Read the model definition and answer for the solid it produces. Units are mm, in the model's axes. A direction names the side the tool comes from. Coordinates: 2 decimals unless noted, no trailing zeros. Loops run counter-clockwise (first coordinate to the right, second up) from the corner with the lowest first, then second, coordinate; pieces in that order, holes last. Notation, with made-up numbers: (-26, 73) - (-19, 73) arc R30 ccw to (-19, 99) - close; hole circle Ø6 at (15.5, 73.5). An arc over 180 degrees is marked (long way). Use one line per item in the form item = value.
from build123d import *

# Parameters (mm, degrees)
CROQUIS1_W               = 118
CROQUIS1_H               = 74
SALIENTE_EXTRUIR1_DEPTH  = 5
CROQUIS2_W               = 50
CROQUIS2_H               = 40
CORTAR_EXTRUIR1_DEPTH    = 5
CROQUIS3_W               = 50
CROQUIS3_H               = 5
SALIENTE_EXTRUIR2_DEPTH  = 3
CROQUIS4_W               = 4.8
CROQUIS4_H               = 2.8
CROQUIS4_W_2             = 2.8
CROQUIS4_H_2             = 4.8
CORTAR_EXTRUIR2_DEPTH    = 6
CROQUIS5_W               = 3
CROQUIS5_H               = 40
CORTAR_EXTRUIR3_DEPTH    = 3
CROQUIS6_W               = 12
CROQUIS6_H               = 40
SALIENTE_EXTRUIR3_DEPTH  = 40
CROQUIS8_W               = 4
CROQUIS8_H               = 35
SALIENTE_EXTRUIR5_DEPTH  = 5
SALIENTE_EXTRUIR7_DEPTH  = 33
CORTAR_EXTRUIR6_DEPTH    = 11
CORTAR_EXTRUIR7_DEPTH    = 13
CORTAR_EXTRUIR8_DEPTH    = 13
CORTAR_EXTRUIR9_DEPTH    = 11
CROQUIS10_W              = 1.9
CROQUIS10_H              = 35
SALIENTE_EXTRUIR9_DEPTH  = 8
CROQUIS22_W              = 3.1
CROQUIS22_H              = 35
SALIENTE_EXTRUIR10_DEPTH = 2
CORTAR_EXTRUIR11_DEPTH   = 40
CROQUIS23_W              = 3
CROQUIS23_H              = 40
SALIENTE_EXTRUIR11_DEPTH = 10
CORTAR_EXTRUIR12_DEPTH   = 10
CORTAR_EXTRUIR13_DEPTH   = 10
CORTAR_EXTRUIR14_DEPTH   = 40
CROQUIS28_R              = 1.25
CORTAR_EXTRUIR15_DEPTH   = 5
SALIENTE_EXTRUIR12_DEPTH = 37
CROQUIS30_W              = 29.42787794
CROQUIS30_H              = 11
SALIENTE_EXTRUIR13_DEPTH = 1.970920231
CHAFL_N1_SIZE            = 5
CHAFL_N1_SIZE2           = 18
CHAFL_N2_SIZE            = 5
CHAFL_N2_SIZE_2          = 13
CHAFL_N3_SIZE            = 5
CHAFL_N3_SIZE_2          = 13
CROQUIS51_W              = 8
CROQUIS51_H              = 14
CORTAR_EXTRUIR23_DEPTH   = 10
CROQUIS52_W              = 9
CROQUIS52_H              = 11
CROQUIS52_W_2            = 8
CROQUIS52_W_3            = 4.539822883
CORTAR_EXTRUIR25_DEPTH   = 10
SALIENTE_EXTRUIR20_DEPTH = 12
CROQUIS54_W              = 5
CROQUIS54_H              = 11
CORTAR_EXTRUIR26_DEPTH   = 10
CROQUIS55_W              = 5
CROQUIS55_H              = 11
CORTAR_EXTRUIR30_DEPTH   = 10


with BuildPart() as part:
    # Croquis1 → Saliente-Extruir1 (new body)
    with BuildSketch(Plane.XY):
        Rectangle(CROQUIS1_W, CROQUIS1_H)
    extrude(amount=SALIENTE_EXTRUIR1_DEPTH)

    # Croquis2 → Cortar-Extruir1 (cut)
    with BuildSketch(Plane.XY.offset(5)):
        with Locations((-21, 0)):
            Rectangle(CROQUIS2_W, CROQUIS2_H)
    extrude(amount=-CORTAR_EXTRUIR1_DEPTH, mode=Mode.SUBTRACT)

    # Croquis3 → Saliente-Extruir2 (add)
    with BuildSketch(Plane.XY.offset(5)):
        with Locations((34, 34.5)):
            Rectangle(CROQUIS3_W, CROQUIS3_H)
        with Locations((34, -34.5)):
            Rectangle(CROQUIS3_W, CROQUIS3_H)
    extrude(amount=SALIENTE_EXTRUIR2_DEPTH)

    # Croquis4 → Cortar-Extruir2 (cut)
    with BuildSketch(Plane.XY.offset(8)):
        with Locations((54.5, 34.5)):
            Rectangle(CROQUIS4_W, CROQUIS4_H)
        with Locations((12.5, 34.5)):
            Rectangle(CROQUIS4_W, CROQUIS4_H)
        with Locations((12.5, -34.5)):
            Rectangle(CROQUIS4_W, CROQUIS4_H)
        with Locations((54.5, -34.5)):
            Rectangle(CROQUIS4_W, CROQUIS4_H)
        with Locations((-56.5, -32.5)):
            Rectangle(CROQUIS4_W_2, CROQUIS4_H_2)
        with Locations((-56.5, 32.5)):
            Rectangle(CROQUIS4_W_2, CROQUIS4_H_2)
    extrude(amount=-CORTAR_EXTRUIR2_DEPTH, mode=Mode.SUBTRACT)

    # Croquis5 → Cortar-Extruir3 (cut)
    with BuildSketch(Plane.XY.offset(5)):
        with Locations((39.5, 0)):
            Rectangle(CROQUIS5_W, CROQUIS5_H)
    extrude(amount=-CORTAR_EXTRUIR3_DEPTH, mode=Mode.SUBTRACT)

    # Croquis6 → Saliente-Extruir3 (add)
    with BuildSketch(Plane.XY.offset(2)):
        with Locations((47, 0)):
            Rectangle(CROQUIS6_W, CROQUIS6_H)
    extrude(amount=SALIENTE_EXTRUIR3_DEPTH)

    # Croquis8 → Saliente-Extruir5 (add)
    with BuildSketch(Plane.XY.offset(5)):
        with Locations((15, 0)):
            Rectangle(CROQUIS8_W, CROQUIS8_H)
    extrude(amount=SALIENTE_EXTRUIR5_DEPTH)

    # Croquis12 → Saliente-Extruir7 (add)
    with BuildSketch(Plane.XY.offset(5)):
        Polygon((26, -19), (38, -19), (38, -32), (31, -32), (31, -21), (26, -21), align=None)
        Polygon((31, 32), (38, 32), (38, 19), (26, 19), (26, 21), (31, 21), align=None)
    extrude(amount=SALIENTE_EXTRUIR7_DEPTH)

    # Croquis14 → Cortar-Extruir6 (cut)
    with BuildSketch(Plane(origin=(0, 32, 0), x_dir=(1, 0, 0), z_dir=(0, 1, 0))):
        Polygon((31, -38), (36, -38), (31, -9), align=None)
    extrude(amount=-CORTAR_EXTRUIR6_DEPTH, mode=Mode.SUBTRACT)

    # Croquis16 → Cortar-Extruir7 (cut)
    with BuildSketch(Plane.XZ.offset(-19)):
        Polygon((38, 38), (38, 5), (33, 5), (33, 9), align=None)
    extrude(amount=-CORTAR_EXTRUIR7_DEPTH, mode=Mode.SUBTRACT)

    # Croquis17 → Cortar-Extruir8 (cut)
    with BuildSketch(Plane.XZ.offset(32)):
        Polygon((38, 38), (38, 5), (33, 5), (33, 9), align=None)
    extrude(amount=-CORTAR_EXTRUIR8_DEPTH, mode=Mode.SUBTRACT)

    # Croquis18 → Cortar-Extruir9 (cut)
    with BuildSketch(Plane.XZ.offset(32)):
        Polygon((31, 38), (36, 38), (31, 9), align=None)
    extrude(amount=-CORTAR_EXTRUIR9_DEPTH, mode=Mode.SUBTRACT)

    # Croquis10 → Saliente-Extruir9 (add)
    with BuildSketch(Plane.ZY.offset(-13)):
        with Locations((9.05, 0)):
            Rectangle(CROQUIS10_W, CROQUIS10_H)
    extrude(amount=SALIENTE_EXTRUIR9_DEPTH)

    # Croquis22 → Saliente-Extruir10 (add)
    with BuildSketch(Plane.ZY.offset(-13)):
        with Locations((6.55, 0)):
            Rectangle(CROQUIS22_W, CROQUIS22_H)
    extrude(amount=SALIENTE_EXTRUIR10_DEPTH)

    # Croquis7 → Cortar-Extruir11 (cut)
    with BuildSketch(Plane.XZ.offset(20)):
        Polygon((51.717967697, 42), (41, 2), (41, 42), align=None)
    extrude(amount=-CORTAR_EXTRUIR11_DEPTH, mode=Mode.SUBTRACT)

    # Croquis23 → Saliente-Extruir11 (add)
    with BuildSketch(Plane(origin=(38, 0, 0), x_dir=(0, 0, -1), z_dir=(1, 0, 0))):
        with Locations((-3.5, 0)):
            Rectangle(CROQUIS23_W, CROQUIS23_H)
    extrude(amount=SALIENTE_EXTRUIR11_DEPTH)

    # Croquis25 → Cortar-Extruir12 (cut)
    with BuildSketch(Plane.XZ.offset(20)):
        Polygon((53, 42), (53, 5), (46, 5), align=None)
    extrude(amount=-CORTAR_EXTRUIR12_DEPTH, mode=Mode.SUBTRACT)

    # Croquis26 → Cortar-Extruir13 (cut)
    with BuildSketch(Plane(origin=(0, 20, 0), x_dir=(1, 0, 0), z_dir=(0, 1, 0))):
        Polygon((53, -5), (53, -42), (46, -5), align=None)
    extrude(amount=-CORTAR_EXTRUIR13_DEPTH, mode=Mode.SUBTRACT)

    # Croquis27 → Cortar-Extruir14 (cut)
    with BuildSketch(Plane.XZ.offset(20)):
        Polygon((51.717967697, 42), (53, 42), (53, 41.49489384), align=None)
    extrude(amount=-CORTAR_EXTRUIR14_DEPTH, mode=Mode.SUBTRACT)

    # Croquis28 → Cortar-Extruir15 (cut)
    with BuildSketch(Plane(origin=(37.753520778, 0, -10.116025404), x_dir=(0.25881904510251397, 0, 0.9659258262890701), z_dir=(-0.9659258262890701, 0, 0.25881904510251397))):
        with Locations((20.801870381, 14)):
            Circle(CROQUIS28_R)
        with Locations((48.801870381, 14)):
            Circle(CROQUIS28_R)
        with Locations((48.801870381, -14)):
            Circle(CROQUIS28_R)
        with Locations((20.801870381, -14)):
            Circle(CROQUIS28_R)
    extrude(amount=-CORTAR_EXTRUIR15_DEPTH, mode=Mode.SUBTRACT)

    # Croquis29 → Saliente-Extruir12 (add)
    with BuildSketch(Plane(origin=(59, 0, 0), x_dir=(0, 0, -1), z_dir=(1, 0, 0))):
        Polygon((-8, 37), (0, 37), (0, -37), (-8, -37), (-8, -32), (-5, -32), (-5, 32), (-8, 32), align=None)
    extrude(amount=SALIENTE_EXTRUIR12_DEPTH)

    # Croquis30 → Saliente-Extruir13 (add)
    with BuildSketch(Plane(origin=(28.598152425, 0, -4.930715935), x_dir=(0.1699069165076461, 0, 0.9854601157443481), z_dir=(-0.9854601157443481, 0, 0.1699069165076461))):
        with Locations((28.850194423, 26.5)):
            Rectangle(CROQUIS30_W, CROQUIS30_H)
    saliente_extruir13 = extrude(amount=-SALIENTE_EXTRUIR13_DEPTH)

    # Simetría3: Saliente-Extruir13 across plane
    add(saliente_extruir13.mirror(Plane.ZX))

    # Chaflán1
    chafl_n1_edges = [part.edges().sort_by_distance(p)[0] for p in [
        (53, 0, 5),
    ]]
    chafl_n1_side = [part.faces().sort_by_distance(p)[0] for p in [
        (23.870652036, 0, 5),
    ]]
    chamfer(chafl_n1_edges, length=CHAFL_N1_SIZE, length2=CHAFL_N1_SIZE2, reference=chafl_n1_side[0])

    # Chaflán2
    # the kernel refuses this chamfer: 13, 5 mm, written as the material it adds along each edge
    with BuildSketch(Plane(origin=(33, 19, 5), x_dir=(0.9956504543602249, 0, -0.09316744459454417), z_dir=(0, 1, 0))) as chafl_n2_piece_1:
        Polygon((CHAFL_N2_SIZE * 0.99565045436, -CHAFL_N2_SIZE * 0.0931674445945), (-CHAFL_N2_SIZE_2 * 0.0931674445945, -CHAFL_N2_SIZE_2 * 0.99565045436), (0, 0), align=None)
    extrude(amount=13)

    # Chaflán3
    # the kernel refuses this chamfer: 13, 5 mm, written as the material it adds along each edge
    with BuildSketch(Plane(origin=(33, -32, 5), x_dir=(0.9956504543602249, 0, -0.09316744459454485), z_dir=(0, 1, 0))) as chafl_n3_piece_1:
        Polygon((CHAFL_N3_SIZE * 0.99565045436, -CHAFL_N3_SIZE * 0.0931674445945), (-CHAFL_N3_SIZE_2 * 0.0931674445945, -CHAFL_N3_SIZE_2 * 0.99565045436), (0, 0), align=None)
    extrude(amount=13)

    # Croquis51 → Cortar-Extruir23 (cut)
    with BuildSketch(Plane(origin=(37.753520778, 0, -10.116025404), x_dir=(0.2588190451025144, 0, 0.96592582628907), z_dir=(-0.96592582628907, 0, 0.2588190451025144))):
        with Locations((49.954479718, 0.233117344)):
            Rectangle(CROQUIS51_W, CROQUIS51_H)
    extrude(amount=-CORTAR_EXTRUIR23_DEPTH, mode=Mode.SUBTRACT)

    # Croquis52 → Cortar-Extruir25 (cut)
    with BuildSketch(Plane(origin=(28.598152425, 0, -4.930715935), x_dir=(0.1699069165076461, 0, 0.985460115744348), z_dir=(-0.985460115744348, 0, 0.1699069165076461))):
        with Locations((19.69441499, -26.5)):
            Rectangle(CROQUIS52_W, CROQUIS52_H)
        with Locations((33.19441499, -26.5)):
            Rectangle(CROQUIS52_W_2, CROQUIS52_H)
        with Locations((43.464326432, -26.5)):
            Rectangle(CROQUIS52_W_3, CROQUIS52_H)
    cortar_extruir25 = extrude(amount=-CORTAR_EXTRUIR25_DEPTH, mode=Mode.SUBTRACT)

    # Croquis53 → Saliente-Extruir20 (add)
    with BuildSketch(Plane.XZ.offset(32)):
        Polygon((31, 9), (30.122515807, 3.910591681), (31.179788624, 3.910591681), align=None)
    saliente_extruir20 = extrude(amount=-SALIENTE_EXTRUIR20_DEPTH)

    # Simetría8: Cortar-Extruir25, Saliente-Extruir20 across plane
    add(cortar_extruir25.mirror(Plane.ZX), mode=Mode.SUBTRACT)
    add(saliente_extruir20.mirror(Plane.ZX))

    # Croquis54 → Cortar-Extruir26 (cut)
    with BuildSketch(Plane(origin=(28.598152425, 0, -4.930715935), x_dir=(0.16990691650764617, 0, 0.985460115744348), z_dir=(-0.985460115744348, 0, 0.16990691650764617))):
        with Locations((26.69441499, 26.5)):
            Rectangle(CROQUIS54_W, CROQUIS54_H)
    extrude(amount=-CORTAR_EXTRUIR26_DEPTH, mode=Mode.SUBTRACT)

    # Croquis55 → Cortar-Extruir30 (cut)
    with BuildSketch(Plane(origin=(28.598152425, 0, -4.930715935), x_dir=(0.16990691650764617, 0, 0.985460115744348), z_dir=(-0.985460115744348, 0, 0.16990691650764617))):
        with Locations((26.69441499, -26.5)):
            Rectangle(CROQUIS55_W, CROQUIS55_H)
    extrude(amount=-CORTAR_EXTRUIR30_DEPTH, mode=Mode.SUBTRACT)


solid = part.part
Item 1: For a pull along X with two mould halves and no side action, classify faces 6 (the flat face through (11, 0, 7)), 7 (the flat face through (33.757, -26.577, 9.598)), 8 (the flat face through (12, 35, 2)), 9 (the flat face through (36.9, 23.06, 31.62)) as +X half, -X half, draft (parallel to the pull), parting line (faces both ways), or undercut.
Results below:
face_6 = -X half
face_7 = +X half
face_8 = undercut
face_9 = undercut
Item 2: The part is cut by section C-C on z = 25.5. Give the vertices of the cut face in (x, y), plus the area to 3 significant figures.
Results below:
outline = (26, -21) - (35.84, -21) - (35.84, -19) - (26, -19) - close; (26, 19) - (35.84, 19) - (35.84, 21) - (26, 21) - close; (47.3, -20) - (49.88, -20) - (49.88, -10) - (53, -10) - (53, 10) - (49.88, 10) - (49.88, 20) - (47.3, 20) - close
area = 205 mm²
Item 3: Each of these flat-tipped pins is pushed along its axis until it touches: P1, Ø2, axis at x = -6, y = -26.5, coming from the -Z side; P2, Ø2, axis at x = 53.5, y = -34, coming from the +Z side; P3, Ø1.5, axis at y = -8, z = 29, coming from the -X side; P4, Ø8, axis at x = 48, z = 34.5, coming from the +Y side. Where does it stop, or does it pass through?
Results below:
P1 = 0
P2 = 8
P3 = 48.03
P4 = 20
Item 4: The part is cut by section A-A on y = 22.5. Give the vertices of the cut face in (x, z), plus the area to 3 significant figures.
Results below:
outline = (-59, 0) - (96, 0) - (96, 5) - (38, 5) - (36.41, 9.14) - (31.18, 10.04) - (30.31, 5) - (-59, 5) - close; (34.92, 31.72) - (36.86, 31.39) - (37.54, 35.33) - (35.6, 35.66) - close
area = 812 mm²
Item 5: The part is cut by section D-D on x = 65.5. Give the vertices of the cut face in (y, z), plus the area to 3 significant figures.
Results below:
outline = (-37, 0) - (37, 0) - (37, 8) - (32, 8) - (32, 5) - (-32, 5) - (-32, 8) - (-37, 8) - close
area = 400 mm²
Item 6: Find the intervals of material crossed by L1, parallel to X at y = 2, z = 2.5; L2, parallel to Y at x = -14.5, z = 4.5; L3, parallel to Z at x = -50, y = 27, in increasing order.
Results below:
L1 = -59 to -46, 4 to 96
L2 = -37 to -20, 20 to 37
L3 = 0 to 5
Item 7: The part is cut by section B-B on x = -6. Give the vertices of the cut face in (y, z).
Results below:
outline = (-37, 0) - (-20, 0) - (-20, 5) - (-37, 5) - close; (20, 0) - (37, 0) - (37, 5) - (20, 5) - close
Item 8: Which of the six approach directions +Z, -Z, +X, -X, +Y, -Y give full straight-line access (tool end or side, diameter ignored) to faces 1 (the flat face through (-57, 33, 2)), 2 (the flat face through (12, -17.5, 8)), 3 (the flat face through (35.262, -26.577, 33.721)), 4 (the flat face through (-59, -1, 2)), 5 (the flat face through (9, 34, 6))?
Results below:
face_1 = +Z
face_2 = +Z, -X
face_3 = +Z, -X, -Y
face_4 = +Z, -Z, -X, +Y, -Y
face_5 = +Z, -X, +Y, -Y
